Read the model definition and answer for the solid it produces. Units are mm, in the model's axes. Coordinates: 2 decimals unless noted, no trailing zeros. Loops run counter-clockwise (first coordinate to the right, second up) from the corner with the lowest first, then second, coordinate; pieces in that order, holes last.
from build123d import *

# Parameters (mm, degrees)
BOSS_EXTRUDE1_DEPTH = 3
SKETCH2_R           = 2.25
CUT_EXTRUDE1_DEPTH  = 7.806859286
FILLET1_R           = 0.5
SWEEP3_PITCH        = 0.5


with BuildPart() as part:
    # Sketch1 → Boss-Extrude1 (new body)
    with BuildSketch(Plane(origin=(0, 0, 0), x_dir=(1, 0, 0), z_dir=(0, 1, 0))):
        Polygon((2.309401077, -4), (4.618802154, 0), (2.309401077, 4), (-2.309401077, 4), (-4.618802154, 0), (-2.309401077, -4), align=None)
    extrude(amount=BOSS_EXTRUDE1_DEPTH)

    # Sketch2 → Cut-Extrude1 (cut, through all)
    with BuildSketch(Plane(origin=(0, 3, 0), x_dir=(1, 0, 0), z_dir=(0, 1, 0))):
        with Locations(Location((0, 0, 0), (0, 0, 270))):
            Circle(SKETCH2_R)
    extrude(amount=-CUT_EXTRUDE1_DEPTH, mode=Mode.SUBTRACT)

    # Fillet1
    fillet1_edges = [part.edges().sort_by_distance(p)[0] for p in [
        (-2.309401077, 1.5, 4),
        (-4.618802154, 1.5, 0),
        (-2.309401077, 1.5, -4),
        (2.309401077, 1.5, -4),
        (4.618802154, 1.5, 0),
        (2.309401077, 1.5, 4),
    ]]
    fillet(fillet1_edges, radius=FILLET1_R)

    # Sweep3: the profile of Sketch5 profile screwed along a left-hand helix of 6 turns, 6 arcs to a turn; built about Z, then put on its axis
    sweep3_z = Axis((0, 0, 0), (0, 0, 1))
    sweep3_corners = [(2.2503, 0, 0.225173205), (1.860288568, 0, 0), (2.2503, 0, -0.225173205)]
    with BuildLine(mode=Mode.PRIVATE) as sweep3_profile:
        Line(sweep3_corners[0], sweep3_corners[1])
        Line(sweep3_corners[1], sweep3_corners[2])
        Line(sweep3_corners[2], sweep3_corners[0])
    sweep3_cap = Face(sweep3_profile.wire())
    sweep3_turn_angles = [0, -30, -60, -90, -120, -150, -180, -210, -240, -270, -300, -330, -360]
    sweep3_turn_weights = [1, 0.8660254037844387, 1, 0.8660254037844387, 1, 0.8660254037844387, 1, 0.8660254037844387, 1, 0.8660254037844387, 1, 0.8660254037844387, 1]
    sweep3_turn_rails = [Edge.make_bspline([Vector(p[0], p[1], 0).rotate(sweep3_z, sweep3_turn_angles[k]) / sweep3_turn_weights[k] + Vector(0, 0, p[2] + -SWEEP3_PITCH * sweep3_turn_angles[k] / 360) for k in range(13)], [0, 0, 0, 1, 1, 2, 2, 3, 3, 4, 4, 5, 5, 6, 6, 6], 2, sweep3_turn_weights) for p in sweep3_corners]
    sweep3_turn_sides = [Face.make_surface_from_curves(sweep3_turn_rails[p[0]], sweep3_turn_rails[p[1]]) for p in [(0, 1), (1, 2), (2, 0)]]
    sweep3 = Plane(origin=(0, 3, 0), x_dir=(0, 0, 1), z_dir=(0, -1, 0)) * Solid(Shell([*[p.moved(Location((0, 0, SWEEP3_PITCH * i))) for i in range(6) for p in sweep3_turn_sides], sweep3_cap, sweep3_cap.rotate(sweep3_z, -2160).moved(Location((0, 0, -SWEEP3_PITCH * -2160 / 360)))]))
    add(sweep3)

    # SurfaceCut1
    split(bisect_by=Plane(origin=(0, 3, 0), x_dir=(1, 0, 0), z_dir=(0, 1, 0)), keep=Keep.BOTTOM)

    # SurfaceCut2
    split(bisect_by=Plane(origin=(0, 0, 0), x_dir=(-1, 0, 0), z_dir=(0, -1, 0)), keep=Keep.BOTTOM)


solid = part.part
Item 1: Find the intervals of material crossed by line 1 along Z through (x, y) = (1, 2.35); line 2 along Z through (x, y) = (0, 0.55); line 3 along Z through (x, y) = (4, 1.35), in increasing order.
Numbers:
line 1: z = -4 to -1.69, 1.79 to 4
line 2: z = -4 to -2.21, 1.95 to 4
line 3: z = -1.07 to 1.07
Item 2: A cutting plane is placed at A-A on z = 3.25. Determine the outline of the cut face in (x, y).
Numbers:
outline: (-2.74, 0) - (2.74, 0) - (2.74, 3) - (-2.74, 3) - close
Item 3: A cutting plane is placed at C-C on z = 2. Give the number of separate pieces and of enclosed holes in the cut face, then the cut area to 3 significant figures.
Numbers:
separate pieces: 1
enclosed holes: 4
area: 17.6 mm2
Item 4: Given pin 1 (2.5 mm diameter, centred on x = 0, z = 0, fed in from -Y), flat-ended and moving along its own axis, determine where the tip first touches the part or whether it passes through.
Numbers:
pin 1: passes through
Item 5: A cutting plane is placed at B-B on x = 3.5. Determine the outline of the cut face in (y, z), then the cut area to 3 significant figures.
Numbers:
outline: (0, -1.94) - (3, -1.94) - (3, 1.94) - (0, 1.94) - close
area: 11.6 mm2
